Here's how the part is built. I have some questions about the finished solid (model axes, mm). A direction names the side the tool comes from. Round coordinates to 2 decimals unless told otherwise and drop trailing zeros. Order: outer loops, then holes, each group sorted by start corner. A loop starts at its lowest first (then second) coordinate and runs counter-clockwise, first axis right, second up. Notation, with made-up numbers: (5, -25.75) -> (49, -25.75) arc R20 cw to (49, 3.25) -> close; hole circle Ø2 at (-27.75, -9). An arc over 180 degrees is marked (long way). One line per item, written item: value.
Autodesk Inventor part; units mm, degrees
ref_plane "YZ Plane" through (0, 0, 0) normal (1, 0, 0) x (0, 1, 0)
ref_plane "XZ Plane" through (0, 0, 0) normal (0, 1, 0) x (-1, 0, 0)
ref_plane "XY Plane" through (0, 0, 0) normal (0, 0, 1) x (1, 0, 0)
sketch "Sketch1" plane through (-152.4, -88.9, 0) normal (0, 0, 1) x (1, 0, 0)
  line L0 (2.3554, 30.5524) -> (256.3554, 30.5524)
  line L1 (256.3554, 30.5524) -> (256.3554, 157.5524)
  line L2 (256.3554, 157.5524) -> (2.3554, 157.5524)
  line L3 (2.3554, 157.5524) -> (2.3554, 30.5524)
  line L4 (-16.6946, 30.5524) -> (275.4054, 30.5524)
  line L5 (275.4054, 30.5524) -> (275.4054, 176.6024)
  line L6 (275.4054, 176.6024) -> (-16.6946, 176.6024)
  line L7 (-16.6946, 176.6024) -> (-16.6946, 30.5524)
  point P0 (129.3554, 30.5524)
  point P1 (256.3554, 30.5524)
  point P2 (2.3554, 30.5524)
  dimension "d2" = 254
  dimension "d3" = 127
  dimension "d0" = 19.05
  dimension "d1" = 19.05
extrude "Extrusion1" add sketch "Sketch1" along normal blind 12.7 contours L4 L7 L6 L5 L1 L2 L3
extrude "Extrusion2" add sketch "Sketch1" along normal blind 9.525 contours L3 L2 L1 L0
chamfer "Chamfer1" distance 10.16 angle 45 3 edges at (-169.0946, 14.6774, 12.7) (-23.0446, 87.7024, 12.7) (123.0054, 14.6774, 12.7)
ref_plane "Work Plane1" through (-169.0946, 87.7024, 0) normal (1, 0, 0) x (0, -1, 0)
sketch "Sketch2" plane through (-169.0946, 87.7024, 0) normal (1, 0, 0) x (0, -1, 0)
  line L0 (0, 0) -> (146.05, 0)
  point P0 (88.9, 0)
  point P1 (88.9, 0)
  dimension "d17" = 88.9
ref_plane "Work Plane2" through (123.0054, 87.7024, 0) normal (0, -1, 0) x (-1, 0, 0)
equation "\"d1\" = d0"
properties part number "Top Base"
Q1. For P1, Ø1.6, axis at y = 5, z = 10.5, coming from the -X side; P2, Ø1, axis at y = 7.5, z = 5, coming from the +X side; P3, Ø6, axis at y = -4, z = 8, coming from the +X side; P4, Ø6, axis at x = -94, z = 4.5, coming from the +Y side, each with a flat end and sliding along its axis, tell me the tip position at first contact or that it passes through.
Answers:
P1: x = -161.93
P2: x = 121.05
P3: x = 120.55
P4: y = 87.7
Q2. Which directions (+Z, -Z, +X, -X, +Y, -Y) give clear straight access to the entire face, cutting with the end or side of a thin tool? Please do faces 1 (the face through (-21, 82.69, 7.55)), 2 (the face through (-25, 6, 9.525)).
Answers:
face 1: +Z, +X, -X, +Y
face 2: +Z, -Y
Q3. I need wall thicknesses on line 1 along Z through (x, y) = (2, 49) (3 decimals); line 2 along X through (y, z) = (-47, 10.25); line 3 along X through (y, z) = (-34, 11.25). Which ranges of each line are inside material? Lowest first, please.
Answers:
line 1: 0 to 9.525
line 2: -161.38 to -150.04, 103.96 to 115.3
line 3: -160.38 to -150.04, 103.96 to 114.3
Q4. I want a section at A-A on y = -20. Write out the boundary of the cut face in (x, z) (3 decimals), then the cut area to 3 significant figures.
Answers:
outline: (-169.095, 0) -> (123.005, 0) -> (123.005, 2.54) -> (112.845, 12.7) -> (103.955, 12.7) -> (103.955, 9.525) -> (-150.045, 9.525) -> (-150.045, 12.7) -> (-158.935, 12.7) -> (-169.095, 2.54) -> close
area: 2,800 mm2
Q5. I want a section at B-B on x = -97. Write out the boundary of the cut face in (y, z) (3 decimals).
Answers:
outline: (-58.348, 0) -> (87.702, 0) -> (87.702, 2.54) -> (77.542, 12.7) -> (68.652, 12.7) -> (68.652, 9.525) -> (-58.348, 9.525) -> close
Q6. I want a section at C-C on z = 6.25. Write out the boundary of the cut face in (x, y).
Answers:
outline: (-165.38, -58.35) -> (119.3, -58.35) -> (119.3, 83.99) -> (-165.38, 83.99) -> close
